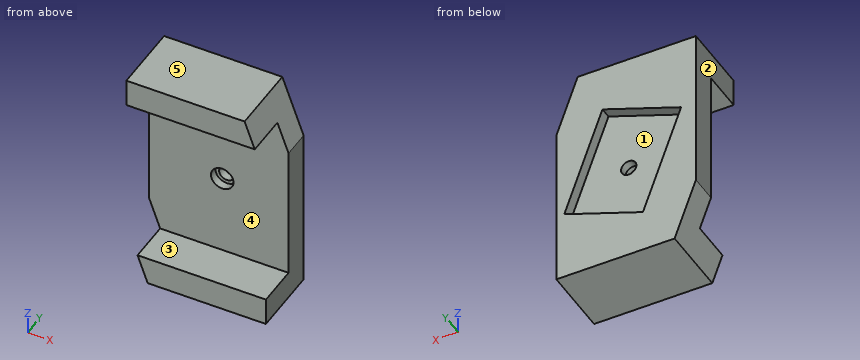
Autodesk Inventor part; units mm, degrees
ref_plane "Work Plane1" through (25.25, 0, 0) normal (1, 0, 0) x (0, 1, 0)
ref_plane "Work Plane2" through (0, 25, 0) normal (0, 1, 0) x (-1, 0, 0)
ref_plane "Work Plane3" through (0, 21, 0) normal (0, 1, 0) x (-1, 0, 0)
sketch "Sketch1" plane through (0, 0, 0) normal (0, 1, 0) x (-1, 0, 0)
  line L0 (-25, -40) -> (25, -40) construction
  line L1 (25, -40) -> (25, 40) construction
  line L2 (25, 40) -> (-25, 40) construction
  line L3 (-25, 40) -> (-25, -40) construction
  line L4 (-25, 19) -> (-17.3566, 40)
  line L5 (17.3566, -40) -> (25, -19)
  line L6 (25, -19) -> (25, 40)
  line L7 (25, 40) -> (-17.3566, 40)
  line L8 (-25, 19) -> (-25, -40)
  line L9 (-25, -40) -> (17.3566, -40)
  point P0 (0, 0)
  point P1 (25, 0)
  point P2 (0, -40)
  dimension "d0" = 50
  dimension "d1" = 80
  dimension "d2" = 21
  dimension "d3" = 20
  dimension "d4" = 20
  dimension "d5" = 21
extrude "Extrusion1" add sketch "Sketch1" along normal blind 25
ref_plane "Work Plane1" through (25.25, 0, 0) normal (1, 0, 0) x (0, 1, 0)
sketch "Sketch2" plane through (25.25, 0, 0) normal (1, 0, 0) x (0, 1, 0)
  line L0 (0, 40) -> (0, 19) construction
  line L1 (0, 19) -> (25, 19) construction
  line L2 (25, 40) -> (25, 19) construction
  line L3 (0, 40) -> (25, 40) construction
  line L4 (0, 19) -> (0, -40) construction
  line L5 (0, -40) -> (25, -40) construction
  line L6 (25, 19) -> (25, -40) construction
  line L7 (0, 19) -> (25, 19) construction
  line L8 (0, 30) -> (0, -30)
  line L9 (0, 30) -> (15, 30)
  line L10 (15, 30) -> (15, -30)
  line L11 (15, -30) -> (0, -30)
  point P0 (0, 0)
  dimension "d9" = 60
  dimension "d10" = 10
  dimension "d11" = 15
extrude "Extrusion2" cut sketch "Sketch2" against normal through all
ref_plane "Work Plane2" through (0, 25, 0) normal (0, 1, 0) x (-1, 0, 0)
sketch "Sketch3" plane through (0, 25, 0) normal (0, 1, 0) x (-1, 0, 0)
  line L0 (17.3566, -40) -> (25, -19) construction
  line L1 (25, -19) -> (25, 40) construction
  line L2 (25, 40) -> (-17.3566, 40) construction
  line L3 (-17.3566, 40) -> (-25, 19) construction
  line L4 (-25, 19) -> (-25, -40) construction
  line L5 (-25, -40) -> (17.3566, -40) construction
  line L6 (6.0192, -24.6856) -> (-22.1716, -14.425)
  line L7 (-22.1716, -14.425) -> (-8.4908, 23.1627)
  line L8 (-8.4908, 23.1627) -> (19.7, 12.9021)
  line L9 (19.7, 12.9021) -> (6.0192, -24.6856)
  point P0 (0, 0)
  dimension "d15" = 30
  dimension "d16" = 40
  dimension "d17" = 30
  dimension "d18" = 25
  dimension "d19" = 70
  dimension "d20" = 5.3
extrude "Extrusion3" cut sketch "Sketch3" against normal blind 4
ref_plane "Work Plane3" through (0, 21, 0) normal (0, 1, 0) x (-1, 0, 0)
sketch "Sketch4" plane through (0, 21, 0) normal (0, 1, 0) x (-1, 0, 0)
  line L0 (-22.1716, -14.425) -> (-8.4908, 23.1627) construction
  line L1 (-8.4908, 23.1627) -> (19.7, 12.9021) construction
  line L2 (19.7, 12.9021) -> (6.0192, -24.6856) construction
  line L3 (6.0192, -24.6856) -> (-22.1716, -14.425) construction
  line L4 (17.3566, -40) -> (25, -19) construction
  line L5 (25, -19) -> (25, 40) construction
  line L6 (25, 40) -> (-17.3566, 40) construction
  line L7 (-17.3566, 40) -> (-25, 19) construction
  line L8 (-25, 19) -> (-25, -40) construction
  line L9 (-25, -40) -> (17.3566, -40) construction
  line L10 (-8.0762, -19.5553) -> (5.6046, 18.0324) construction
  line L11 (12.8596, -5.8918) -> (-15.3312, 4.3688) construction
  circle A0 centre (-1.2358, -0.7615) radius 2.75
  point P0 (0, 0)
  dimension "d24" = 5.5
extrude "Extrusion4" cut sketch "Sketch4" against normal through all
sketch "Sketch5" plane through (-25, 15, 30) normal (0, -1, 0) x (1, 0, 0)
  circle A0 centre (26.2358, -30.7615) radius 2.75 construction
  circle A1 centre (26.2358, -30.7615) radius 4.05
  point P0 (25, -30)
  dimension "d27" = 8.1
extrude "Extrusion5" cut sketch "Sketch5" against normal blind 3
properties part number "base_obj3"
Work out the finished part from the listing and answer in its coordinate system (mm). Face numbers are marked on the shaded views. A direction names the side the tool comes from. Coordinates: 2 decimals unless noted, no trailing zeros. Loops run counter-clockwise (first coordinate to the right, second up) from the corner with the lowest first, then second, coordinate; pieces in that order, holes last. Notation, with made-up numbers: M 70.25,-21 L 87.25,-21 A20 cw 87.25,-6 Z; hole C 31.25,78 d2. An arc over 180 degrees is marked long. Answer in a Markdown table with one row per item. Add a question column.
1. A flat-ended cylindrical pin translates along its axis: P1, Ø3, axis at x = -17.5, z = 16, coming from the -Y side. Find the tip coordinate at first contact, or state that the pin passes through.
2. Consider L1, parallel to Z at x = 16, y = 1.5; L2, parallel to Y at x = -8, z = -16; L3, parallel to Y at x = -20, z = 16.5. Determine where each line is inside the solid, lowest interval first.
3. A tool of negligible diameter and unlimited length cuts with its end or side. For the marked faces 4 and 5, from which of +Z, -Z, +X, -X, +Y, -Y can it reach the whole face along a straight path? Write none if from no direction.
4. Find section A-A, the plane y = 8.5. Write down the section's boundary in (x, z), then the cut area to 3 significant figures.
5. Find section B-B, the plane z = -8. Write down the section's boundary in (x, y), then the cut area to 3 significant figures.
6. Find section C-C, the plane x = 7. Write down the section's boundary in (y, z), then the cut area to 3 significant figures.
7. Find section D-D, the plane x = -7. Write down the section's boundary in (y, z).
8. The mould has two halves that part along X. Classify the marked faces 1, 2 and 3: pulls with the +X half, pulls with the -X half, needs draft (parallel to the pull), parting line crosses it, or undercut.
Reported:
| question | item | result |
|---|---|---|
| 1 | P1 | stops at y = 15 |
| 2 | L1 | z = -40 to -30, 30 to 40 |
| 2 | L2 | y = 15 to 21 |
| 2 | L3 | y = 15 to 25 |
| 3 | face 4 | +X, -X, -Y |
| 3 | face 5 | +Z, +X, -X, +Y, -Y |
| 4 | outline | M -25,30 L 21,30 L 17.36,40 L -25,40 Z; M -21,-30 L -17.36,-40 L 25,-40 L 25,-30 Z |
| 4 | area | 884 mm^2 |
| 5 | outline | M -25,15 L 25,15 L 25,25 L 19.83,25 L 19.83,21 L -12.09,21 L -12.09,25 L -25,25 Z |
| 5 | area | 372 mm^2 |
| 6 | outline | M 0,-40 L 25,-40 L 25,-19.95 L 21,-19.95 L 21,22.62 L 25,22.62 L 25,40 L 0,40 L 0,30 L 15,30 L 15,-30 L 0,-30 Z |
| 6 | area | 930 mm^2 |
| 7 | outline | M 0,-40 L 25,-40 L 25,-21.99 L 21,-21.99 L 21,17.52 L 25,17.52 L 25,40 L 0,40 L 0,30 L 15,30 L 15,-30 L 0,-30 Z |
| 8 | face 1 | undercut |
| 8 | face 2 | pulls with the -X half |
| 8 | face 3 | needs draft |
